from build123d import *

# Parameters (mm, degrees)
EXTRUDE_1_DEPTH     = 20
SKETCH_2_R          = 3
CUT_EXTRUDE_1_DEPTH = 20
SKETCH_3_R          = 1.75
CUT_EXTRUDE_2_DEPTH = 27.088377855


with BuildPart() as part:
    # 草图1 → 凸台-拉伸1 (new body)
    with BuildSketch(Plane.XY):
        with BuildLine():
            Line((-33.25, 0), (-18.25, 0))
            ThreePointArc((-18.25, 0), (0, 18.25), (18.25, 0))
            Line((18.25, 0), (33.25, 0))
            Line((33.25, 0), (33.25, 13.52748426))
            ThreePointArc((33.25, 13.52748426), (32.911797538, 15.137216782), (31.954380604, 16.474741552))
            Line((31.954380604, 16.474741552), (22.624644973, 25.035635147))
            ThreePointArc((22.624644973, 25.035635147), (21.371293457, 25.815912507), (19.920264369, 26.088377855))
            Line((19.920264369, 26.088377855), (-19.920264369, 26.088377855))
            ThreePointArc((-19.920264369, 26.088377855), (-21.371293457, 25.815912507), (-22.624644973, 25.035635147))
            Line((-22.624644973, 25.035635147), (-31.954380604, 16.474741552))
            ThreePointArc((-31.954380604, 16.474741552), (-32.911797538, 15.137216782), (-33.25, 13.52748426))
            Line((-33.25, 13.52748426), (-33.25, 0))
        make_face()
    extrude(amount=EXTRUDE_1_DEPTH)

    # 草图2 → 切除-拉伸1 (cut)
    with BuildSketch(Plane(origin=(0, 26.088377855, 0), x_dir=(1, 0, 0), z_dir=(0, 1, 0))):
        with Locations((-25.5, -10)):
            Circle(SKETCH_2_R)
        with Locations((25.5, -10)):
            Circle(SKETCH_2_R)
    extrude(amount=-CUT_EXTRUDE_1_DEPTH, mode=Mode.SUBTRACT)

    # 草图3 → 切除-拉伸2 (cut, through all)
    with BuildSketch(Plane(origin=(0, 26.088377855, 0), x_dir=(1, 0, 0), z_dir=(0, 1, 0))):
        with Locations((25.5, -10)):
            Circle(SKETCH_3_R)
        with Locations((-25.5, -10)):
            Circle(SKETCH_3_R)
    extrude(amount=-CUT_EXTRUDE_2_DEPTH, mode=Mode.SUBTRACT)


solid = part.part
Geometry check sheet. Reference: the model listing, model coordinates, mm. A direction names the side the tool comes from. Round coordinates to 2 decimals unless told otherwise and drop trailing zeros. Loops run counter-clockwise (first coordinate to the right, second up) from the corner with the lowest first, then second, coordinate; pieces in that order, holes last. Notation, with made-up numbers: (28, 81.5) -> (52, 81.5) arc R9 cw to (52, 86.5) -> close; hole circle Ø5 at (-16.5, -24). An arc over 180 degrees is marked (long way). Answer as a JSON object with one key per item and string values. Group by question number.
Item 1: Release check for a two-part mould opening along Z. For faces 1 (the face through (0, 19, 0)), 2 (the face through (-28, 0, 10)), 3 (the face through (-26.79, 3.09, 8.82)) record: pulls with the +Z half, pulls with the -Z half, needs draft (parallel to the pull), parting line crosses it, or undercut.
Item 2: Cross-section at A-A, the plane z = 16.5. Record the cut outline in (x, y).
Item 3: Cross-section at B-B, the plane x = 26. Record the cut outline in (y, z).
Item 4: Cross-section at C-C, the plane y = 19. Record the cut outline in (x, z), plus the area to 3 significant figures.
Item 5: Depth check by flat-ended pin: pin 1 Ø3 at (x, z) = (25.5, 9.5) entering from +Y; pin 2 Ø2 at (x, z) = (25.5, 10) entering from +Y; pin 3 Ø9.5 at (x, z) = (-25.5, 10) entering from +Y; pin 4 Ø5 at (y, z) = (20, 6.5) entering from -X. Enter the tip coordinate at first touch or a pass-through.
Item 6: Set-up check for faces 4 (the face through (21.39, 25.81, 9.86)), 5 (the face through (22.5, 13.6, 9.9)): record each of +Z, -Z, +X, -X, +Y, -Y from which the full face is reachable in a straight line by a thin tool's end or side.
Item 7: Cross-section at D-D, the plane z = 10. Record the cut outline in (x, y).
Item 8: Thickness scan on line 1 along X through (y, z) = (13, 10); line 2 along Z through (x, y) = (25.5, 14.5); line 3 along Z through (x, y) = (-25.5, 5.25). Record the ranges inside material, lowest first.
Determined:
{
 "1": {"face 1": "pulls with the -Z half", "face 2": "needs draft", "face 3": "undercut"},
 "2": {"outline": "(-33.25, 0) -> (-18.25, 0) arc R18.25 cw to (18.25, 0) -> (33.25, 0) -> (33.25, 13.53) arc R4 ccw to (31.95, 16.47) -> (22.62, 25.04) arc R4 ccw to (19.92, 26.09) -> (-19.92, 26.09) arc R4 ccw to (-22.62, 25.04) -> (-31.95, 16.47) arc R4 ccw to (-33.25, 13.53) -> close"},
 "3": {"outline": "(0, 0) -> (21.94, 0) -> (21.94, 7.04) -> (6.09, 7.04) -> (6.09, 8.32) -> (0, 8.32) -> close; (0, 11.68) -> (6.09, 11.68) -> (6.09, 12.96) -> (21.94, 12.96) -> (21.94, 20) -> (0, 20) -> close"},
 "4": {"outline": "(-29.2, 0) -> (29.2, 0) -> (29.2, 20) -> (-29.2, 20) -> close; hole circle Ø6 at (-25.5, 10); hole circle Ø6 at (25.5, 10)", "area": "1,110 mm²"},
 "5": {"pin 1": "stops at y = 6.09", "pin 2": "passes through", "pin 3": "stops at y = 26", "pin 4": "stops at x = -30.84"},
 "6": {"face 4": "+Z, -Z, +X, +Y", "face 5": "+Y"},
 "7": {"outline": "(-33.25, 0) -> (-27.25, 0) -> (-27.25, 6.09) -> (-28.5, 6.09) -> (-28.5, 19.64) -> (-31.95, 16.47) arc R4 ccw to (-33.25, 13.53) -> close; (-23.75, 0) -> (-18.25, 0) arc R18.25 cw to (18.25, 0) -> (23.75, 0) -> (23.75, 6.09) -> (22.5, 6.09) -> (22.5, 25.15) arc R4 ccw to (19.92, 26.09) -> (-19.92, 26.09) arc R4 ccw to (-22.5, 25.15) -> (-22.5, 6.09) -> (-23.75, 6.09) -> close; (27.25, 0) -> (33.25, 0) -> (33.25, 13.53) arc R4 ccw to (31.95, 16.47) -> (28.5, 19.64) -> (28.5, 6.09) -> (27.25, 6.09) -> close"},
 "8": {"line 1": "x = -33.25 to -28.5, -22.5 to -12.81, 12.81 to 22.5, 28.5 to 33.25", "line 2": "z = 0 to 7, 13 to 20", "line 3": "z = 0 to 8.25, 11.75 to 20"}
}
